Part model, mm, in its own coordinate system. A direction names the side the tool comes from. Round coordinates to 2 decimals unless told otherwise and drop trailing zeros. Write each loop counter-clockwise with the first axis right and the second up, starting at its lowest first coordinate (ties: lowest second). Pieces come first, ordered by that corner, then holes. Notation, with made-up numbers: M -28.75,-15.5 L 13.25,-15.5 A4 cw 13.25,-11.5 Z; hole C 36.25,60.25 d1. An arc over 180 degrees is marked long. Use one line per item in the form item = value. Start each with the question number.
Item 1: Which spindle directions (+Z, -Z, +X, -X, +Y, -Y) get a long thin tool onto all of the face, cutting with end or side? Do faces 4 (the face through (3.944, -15.037, -12.911)), 5 (the face through (3.944, 12.911, -15.037)), 6 (the face through (3.944, 1.634, 19.816)), 7 (the face through (3.944, 14.149, -10.297)). Say none if no direction does.
Item 2: Cut at B-B, the plane z = 0. Give the cut face in (x, y), then the cut area to 3 significant figures.
Item 3: Mould opens along Z. For faces 1 (the face through (3.944, -10.297, -14.149)), 2 (the face through (3.944, -7.678, -18.341)), 3 (the face through (4.056, -21.728, 3.449)) say: +Z half, -Z half, draft (parallel to the pull), parting line (faces both ways), or undercut.
Item 4: Cut at A-A, the plane y = 0. Give the cut face in (x, z), then the cut area to 3 significant figures.
Item 5: Flat gauge pins, fed straight in: pin 1 Ø5 at (x, z) = (3, 5.5) entering from +Y; pin 2 Ø3 at (y, z) = (-11, 10.5) entering from +X; pin 3 Ø4 at (x, z) = (3.5, -13.5) entering from -Y. Where does each tip first touch, or does it go through?
Item 6: Probe L1, parallel to X at y = 6.25, z = 0; L2, parallel to Z at x = 1.25, y = -17; L3, parallel to X at y = -13, z = 4. List the from-to ranges inside material, lowest first.
Item 7: Cut at C-C, the plane x = 13. Give the cut face in (y, z), then the cut area to 3 significant figures.
from build123d import *

# Parameters (mm, degrees)
BASPROSKE_W           = 8
BASPROSKE_H           = 22
TOOTHCUT_DEPTH        = 33.124756808
TEETHCUTS_COUNT       = 20
TEETHCUTS_ANGLE       = 342
BORSKE_R              = 5
BORE_DEPTH            = 50.0000508
BOSS_EXTRUDE1_START   = 10
SKETCH1_R             = 7
SKETCH1_R_2           = 5
BOSS_EXTRUDE1_DEPTH   = 10
F_5_0MM_DOWEL_HOLE1_D = 5


with BuildPart() as part:
    # BasProSke → Base-Revolve (revolve)
    with BuildSketch(Plane(origin=(0, 0, 0), x_dir=(1, 0, 0), z_dir=(0, 1, 0)), mode=Mode.PRIVATE) as base_revolve_sk:
        with Locations((4, 11)):
            Rectangle(BASPROSKE_W, BASPROSKE_H)
    revolve(base_revolve_sk.sketch.rotate(Axis((-10, 0, 0), (1, 0, 0)), 180), axis=Axis((-10, 0, 0), (1, 0, 0)))

    # TooCutSke → ToothCut (cut, through all)
    with BuildSketch(Plane(origin=(0, 0, 0), x_dir=(0, 0, -1), z_dir=(1, 0, 0))):
        with BuildLine():
            ThreePointArc((0.986171591, 17.471189616), (0, 17.499), (-0.986171591, 17.471189616))
            ThreePointArc((-0.986171591, 17.471189616), (-1.626916196, 19.798789858), (-2.932850173, 21.829260982))
            ThreePointArc((-2.932850173, 21.829260982), (0, 22.0254), (2.932850173, 21.829260982))
            ThreePointArc((2.932850173, 21.829260982), (1.626916196, 19.798789858), (0.986171591, 17.471189616))
        make_face()
    toothcut = extrude(amount=TOOTHCUT_DEPTH, mode=Mode.SUBTRACT)

    # TeethCuts: ToothCut ×20 about axis
    teethcuts_axis = Axis((-10, 0, 0), (1, 0, 0))
    for i in range(1, TEETHCUTS_COUNT):
        add(toothcut.rotate(teethcuts_axis, i * TEETHCUTS_ANGLE / (TEETHCUTS_COUNT - 1)), mode=Mode.SUBTRACT)

    # BorSke → Bore (cut, symmetric)
    with BuildSketch(Plane(origin=(0, 0, 0), x_dir=(0, 0, -1), z_dir=(1, 0, 0))):
        with Locations(Location((0, 0, 0), (0, 0, 180))):
            Circle(BORSKE_R)
    extrude(amount=BORE_DEPTH, both=True, mode=Mode.SUBTRACT)

    # Sketch1 → Boss-Extrude1 (add)
    with BuildSketch(Plane(origin=(8, 0, 0), x_dir=(0, 0, -1), z_dir=(1, 0, 0)).offset(BOSS_EXTRUDE1_START)):
        with Locations(Location((0, 0, 0), (0, 0, 180))):
            Circle(SKETCH1_R)
        Circle(SKETCH1_R_2, mode=Mode.SUBTRACT)
    extrude(amount=-BOSS_EXTRUDE1_DEPTH)

    # 5.0mm Dowel Hole1 (through all)
    with Locations(Plane.XZ.offset(7)):
        with Locations((13, 0)):
            Hole(F_5_0MM_DOWEL_HOLE1_D / 2)


solid = part.part
Model answer:
q1.face_4 = +X, -X, -Y
q1.face_5 = -Z, +X, -X
q1.face_6 = +Z, +X, -X
q1.face_7 = +X, -X
q2.outline = M 0,-17.5 L 8,-17.5 L 8,-7 L 10.5,-7 L 10.5,-5 L 0,-5 Z; M 0,5 L 10.5,5 L 10.5,7 L 8,7 L 8,17.5 L 0,17.5 Z; M 15.5,-7 L 18,-7 L 18,-5 L 15.5,-5 Z; M 15.5,5 L 18,5 L 18,7 L 15.5,7 Z
q2.area = 220 mm²
q3.face_1 = undercut
q3.face_2 = -Z half
q3.face_3 = +Z half
q4.outline = M 0,-17.5 L 8,-17.5 L 8,-7 L 18,-7 L 18,-5 L 0,-5 Z; M 0,5 L 18,5 L 18,7 L 8,7 L 8,17.5 L 0,17.5 Z
q4.area = 240 mm²
q5.pin_1 = 21.79
q5.pin_2 = 8
q5.pin_3 = -15.93
q6.L1 = 0 to 10.5, 15.5 to 18
q6.L2 = -10.33 to -6.7, -4.48 to 4.48, 6.7 to 10.33
q6.L3 = 0 to 8
q7.outline = M -6.54,-2.5 A7 ccw 6.54,-2.5 L 4.33,-2.5 A5 cw -4.33,-2.5 Z; M -6.54,2.5 L -4.33,2.5 A5 cw 4.33,2.5 L 6.54,2.5 A7 ccw Z
q7.area = 54.7 mm²
